Geometry: final body of the model. Coordinates: model frame, mm. Coordinates: 2 decimals unless noted, no trailing zeros. Use CSV: the item, a comma, the result in double quotes. Start each with the question number.
1. Section query A-A on y = -0.55. State how many separate pieces and enclosed holes the cut face has, and give its area (3 significant figures).
2. First-contact query: P1, Ø12, axis at x = 16.5, z = 9.5, coming from the +Y side; P2, Ø0.5, axis at y = -0.5, z = 17.5, coming from the -X side. Flat tips, straight axial feed; report the tip coordinate or a pass-through.
3. Material intervals for line 1 (Z direction, x = -1.5, y = -0.05); line 2 (Z direction, x = 13.5, y = -0.9), sorted ascending.
from build123d import *

# Parameters (mm, degrees)
F0_W     = 2.2
F0_H     = 45.730288
F0_W_2   = 2.1
F1_DEPTH = 1


with BuildPart() as f1:
    # F0 (on Front) → F1 (new body)
    with BuildSketch(Plane.XZ):
        Polygon((-60.96, 27.94), (-63.872576, 27.94), (-63.45094, -27.94), (-60.96, -27.94), (-58.86, -27.94), (-58.8518, -27.94), (-56.678003, -27.94), (-56.678003, -1.502051), (-54.578005, -1.502051), (-54.578005, -27.94), (-52.478005, -27.94), (-50.378005, -27.94), (-48.278005, -27.94), (-48.278005, -1.502051), (-46.378005, -1.502051), (-46.378005, -22.870288), (-46.378005, -27.94), (-44.178005, -27.94), (-41.978005, -27.94), (-39.778005, -27.94), (-39.778005, -1.5), (-37.678009, -1.4986), (-37.678009, -17.679542), (-37.695634, -27.94), (-31.367925, -27.94), (-31.367925, -1.4986), (-29.259725, -1.4986), (-29.259725, -27.94), (-22.957845, -27.94), (-22.957845, -1.4986), (-20.857845, -1.4986), (-20.857845, -27.94), (-14.547765, -27.94), (-14.547765, -1.4986), (-12.447765, -1.4986), (-12.447765, -27.94), (-6.137685, -27.94), (-6.137685, -1.4986), (-4.037685, -1.4986), (-4.037685, -27.94), (4.037685, -27.94), (4.037685, -1.4986), (6.137685, -1.4986), (6.137685, -27.94), (12.447765, -27.94), (12.447765, -1.4986), (14.547765, -1.4986), (14.547765, -27.94), (20.857845, -27.94), (20.857845, -1.4986), (22.957845, -1.4986), (22.957845, -27.94), (29.259725, -27.94), (29.259725, -1.4986), (31.367925, -1.4986), (31.367925, -27.94), (37.695634, -27.94), (37.678009, -17.679542), (37.678009, -1.4986), (39.778005, -1.5), (39.778005, -27.94), (46.378005, -27.94), (46.378005, -1.502051), (48.278005, -1.502051), (48.278005, -27.94), (54.578005, -27.94), (54.578005, -1.502051), (56.678003, -1.502051), (56.678003, -27.94), (62.918797, -27.94), (62.918797, 27.94), (56.678003, 27.94), (56.678003, 1.502051), (54.578005, 1.502051), (54.578005, 27.94), (48.278005, 27.94), (48.278005, 1.502051), (46.378005, 1.502051), (46.378005, 27.94), (39.778005, 27.94), (39.778005, 22.86), (39.778005, 1.502051), (37.678009, 1.502051), (37.695634, 27.94), (31.367925, 27.94), (31.367925, 22.86), (31.367925, 1.502051), (29.259725, 1.502051), (29.259725, 27.94), (22.957845, 27.94), (22.957845, 22.86), (22.957845, 1.502051), (20.857845, 1.502051), (20.857845, 27.94), (14.547765, 27.94), (14.547765, 22.86), (14.547765, 1.502051), (12.447765, 1.502051), (12.447765, 27.94), (6.137685, 27.94), (6.137685, 22.86), (6.137685, 1.502051), (4.037685, 1.502051), (4.037685, 27.94), (-4.037685, 27.94), (-4.037685, 1.502051), (-6.137685, 1.502051), (-6.137685, 22.86), (-6.137685, 27.94), (-12.447765, 27.94), (-12.447765, 1.502051), (-14.547765, 1.502051), (-14.547765, 22.86), (-14.547765, 27.94), (-20.857845, 27.94), (-20.857845, 1.502051), (-22.957845, 1.502051), (-22.957845, 22.86), (-22.957845, 27.94), (-29.259725, 27.94), (-29.259725, 1.502051), (-31.367925, 1.502051), (-31.367925, 22.86), (-31.367925, 27.94), (-34.921541, 27.94), (-37.695634, 27.94), (-37.678009, 1.502051), (-39.778005, 1.502051), (-39.778005, 22.86), (-39.778005, 27.94), (-41.978005, 27.94), (-44.178005, 27.94), (-46.378005, 27.94), (-46.378005, 22.86), (-46.378005, 1.502051), (-48.278005, 1.502051), (-48.278005, 27.94), (-50.378005, 27.94), (-52.478005, 27.94), (-54.578005, 27.94), (-54.578005, 1.502051), (-56.678003, 1.502051), (-56.678003, 19.27661), (-56.678003, 27.94), (-58.7698, 27.94), (-58.86, 27.94), align=None)
        Polygon((-52.478005, 22.86), (-50.378005, 22.86), (-50.378005, -22.870288), (-50.378005, -22.873678), (-52.478005, -22.870288), align=None, mode=Mode.SUBTRACT)
        with Locations((-43.078005, -0.005144)):
            Rectangle(F0_W, F0_H, mode=Mode.SUBTRACT)
        Polygon((-35.572965, 17.750787), (-35.572965, 22.86), (-33.472965, 22.86), (-33.472965, -22.870288), (-35.572965, -22.870288), align=None, mode=Mode.SUBTRACT)
        Polygon((-27.162885, -22.870288), (-27.162885, 17.750787), (-27.162885, 22.86), (-25.062885, 22.86), (-25.062885, -22.870288), align=None, mode=Mode.SUBTRACT)
        Polygon((-18.752805, -22.870288), (-18.752805, 17.750787), (-18.752805, 22.86), (-16.652805, 22.86), (-16.652805, -22.870288), align=None, mode=Mode.SUBTRACT)
        Polygon((-10.342725, -22.870288), (-10.342725, 17.750787), (-10.342725, 22.86), (-8.242725, 22.86), (-8.242725, -22.870288), align=None, mode=Mode.SUBTRACT)
        Polygon((-1.932645, -22.870288), (-1.932645, 17.750787), (-1.932645, 22.86), (0, 22.86), (1.932645, 22.86), (1.932645, 17.750787), (1.932645, -22.870288), (0, -22.870288), align=None, mode=Mode.SUBTRACT)
        Polygon((8.242725, -22.870288), (8.242725, 22.86), (10.342725, 22.86), (10.342725, 17.750787), (10.342725, -22.870288), align=None, mode=Mode.SUBTRACT)
        Polygon((16.652805, 22.86), (18.752805, 22.86), (18.752805, 17.750787), (18.752805, -22.870288), (16.652805, -22.870288), align=None, mode=Mode.SUBTRACT)
        Polygon((25.062885, 22.86), (27.162885, 22.86), (27.162885, 17.750787), (27.162885, -22.870288), (25.062885, -22.870288), align=None, mode=Mode.SUBTRACT)
        Polygon((35.572965, -22.870288), (33.472965, -22.870288), (33.472965, 22.86), (35.572965, 22.86), (35.572965, 17.750787), align=None, mode=Mode.SUBTRACT)
        with Locations((43.078005, -0.005144)):
            Rectangle(F0_W, F0_H, mode=Mode.SUBTRACT)
        with Locations((51.428005, -0.005144)):
            Rectangle(F0_W_2, F0_H, mode=Mode.SUBTRACT)
        Polygon((-60.96, -22.86), (-60.96, 22.86), (-58.778, 22.86), (-58.8518, -22.86), align=None, mode=Mode.SUBTRACT)
        Polygon((58.778, 22.86), (60.96, 22.86), (60.96, -22.86), (58.8518, -22.86), align=None, mode=Mode.SUBTRACT)
    extrude(amount=F1_DEPTH)


solid = f1.part
Results list:
1,separate pieces,"1"
1,enclosed holes,"15"
1,area,"4,010 mm²"
2,P1,"stops at y = 0"
2,P2,"stops at x = -63.8"
3,line 1,"z = -27.94 to -22.87, 22.86 to 27.94"
3,line 2,"z = -1.5 to 1.5"
